Geometry: final body of the model. Coordinates: model frame, mm. Coordinates: 2 decimals unless noted, no trailing zeros. Loops run counter-clockwise (first coordinate to the right, second up) from the corner with the lowest first, then second, coordinate; pieces in that order, holes last. Notation, with made-up numbers: (-2, 6) -> (53, 6) arc R11 ccw to (53, 14) -> close; hole circle Ø2 at (-21.5, 33.5). An arc over 180 degrees is marked (long way). One line per item, written item: value. Start each with the question number.
Item 1: Contact query for a flat-ended pin moving along its axis: pin 1 Ø4 at (x, z) = (-15, -14.175) entering from +Y. Output: stop coordinate, or through.
Item 2: Ray query, probe 1 along Z at (x, y) = (-15, 2.15) (3 decimals); probe 2 along Z at (x, y) = (-15, 0.2) (3 decimals); probe 3 along X at (y, z) = (1.45, 16.5). Return the intervals inside material, ascending. Write a range as from..to.
Item 3: Section query A-A on x = -15. Return loops of the section in (y, z) (3 decimals), then the cut area to 4 significant figures.
Item 4: Section query B-B on y = 1.8. Return loops of the section in (x, z) (3 decimals).
from build123d import *

# Parameters (mm, degrees)
SKETCH1_W           = 34
SKETCH1_H           = 37.25
BOSS_EXTRUDE1_DEPTH = 3
SKETCH2_R           = 2.5
CUT_EXTRUDE1_DEPTH  = 2
SKETCH3_R           = 1.4
CUT_EXTRUDE2_DEPTH  = 2


with BuildPart() as part:
    # Sketch1 → Boss-Extrude1 (new body)
    with BuildSketch(Plane(origin=(0, 0, 0), x_dir=(1, 0, 0), z_dir=(0, 1, 0))):
        Rectangle(SKETCH1_W, SKETCH1_H)
    extrude(amount=BOSS_EXTRUDE1_DEPTH)

    # Sketch2 → Cut-Extrude1 (cut)
    with BuildSketch(Plane(origin=(0, 3, 0), x_dir=(1, 0, 0), z_dir=(0, 1, 0))):
        with Locations((-15, 14.175)):
            Circle(SKETCH2_R)
        with Locations((14.2, -15.825)):
            Circle(SKETCH2_R)
    extrude(amount=-CUT_EXTRUDE1_DEPTH, mode=Mode.SUBTRACT)

    # Sketch3 → Cut-Extrude2 (cut)
    with BuildSketch(Plane(origin=(0, 1, 0), x_dir=(1, 0, 0), z_dir=(0, 1, 0))):
        with Locations((-15, 14.175)):
            Circle(SKETCH3_R)
        with Locations((14.2, -15.825)):
            Circle(SKETCH3_R)
    extrude(amount=-CUT_EXTRUDE2_DEPTH, mode=Mode.SUBTRACT)


solid = part.part
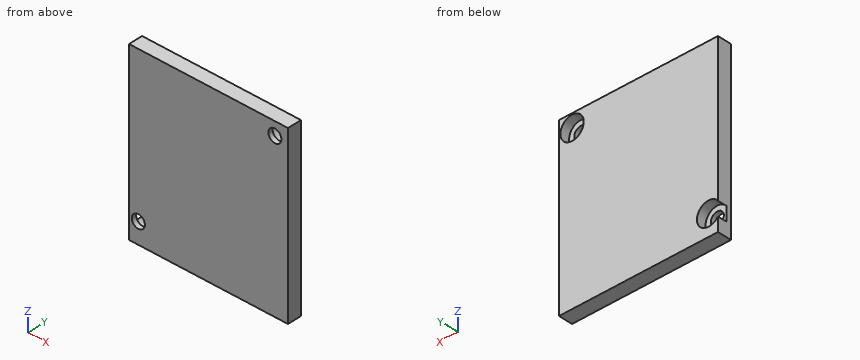
Reply:
1. pin 1: stops at y = 1
2. probe 1: z = -18.625..-16.675, -11.675..18.625
2. probe 2: z = -18.625..-15.575, -12.775..18.625
2. probe 3: x = -17..11.79, 16.61..17
3. outline: (0, -18.625) -> (3, -18.625) -> (3, -16.675) -> (1, -16.675) -> (1, -15.575) -> (0, -15.575) -> close; (0, -12.775) -> (1, -12.775) -> (1, -11.675) -> (3, -11.675) -> (3, 18.625) -> (0, 18.625) -> close
3. area: 98.95 mm²
4. outline: (-17, -18.625) -> (17, -18.625) -> (17, 18.625) -> (-17, 18.625) -> (-17, -12.675) arc R2.5 cw (long way) to (-17, -15.675) -> close; hole circle Ø5 at (14.2, 15.825)
